Verification items for the finished model (mm, model axes). Give positions to 0.01 mm unless a question says otherwise; leave off trailing zeros. Order: outer loops, then holes, each group sorted by start corner. A loop starts at its lowest first (then second) coordinate and runs counter-clockwise, first axis right, second up. Notation, with made-up numbers: (-29.75, -12.5) -> (-2.75, -12.5) arc R32 ccw to (-2.75, 23.5) -> close; hole circle Ø3 at (13, -16.75). An arc over 180 degrees is marked (long way). Write each question's results on one line, items separated by ' | '. Start each with the question number.
1. Cross-section at B-B, the plane y = -30.5. Enter the section's corners in (x, z), then the cut area to 3 significant figures.
2. Cross-section at A-A, the plane z = 1.45. State how many separate pieces and enclosed holes the cut face has, then the cut area to 3 significant figures.
3. Depth check by flat-ended pin: pin 1 Ø5.5 at (x, y) = (-33.34, 52.39) entering from -Z; pin 2 Ø2.5 at (x, z) = (245, 0.5) entering from -Y; pin 3 Ø1.5 at (x, z) = (4, 0) entering from +Y; pin 4 Ø3 at (y, z) = (19, -0.5) entering from +X. Enter the tip coordinate at first touch or a pass-through.
4. Material ranges on L1, parallel to X at y = 41, z = 1.2 (1 decimal); L2, parallel to X at y = 54.5, z = 1.2 (3 decimals); L3, parallel to X at y = 19.5, z = -1.15, recorded low to high. Write a range as from..to.
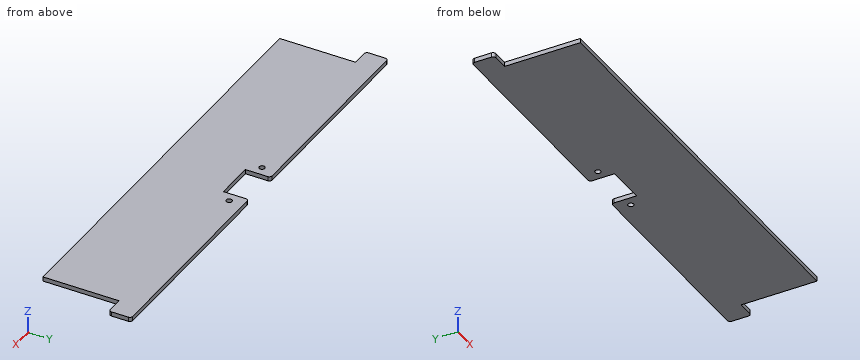
from build123d import *

# Parameters (mm, degrees)
BOSS_EXTRUDE1_DEPTH         = 2.5
SKETCH2_W                   = 44.45
SKETCH2_H                   = 28.575
CUT_EXTRUDE1_DEPTH          = 270.196752221
FILLET1_R                   = 3.175
F_1_4_0_25_DIAMETER_HOLE1_D = 6.35


with BuildPart() as part:
    # Sketch1 → Boss-Extrude1 (new, symmetric)
    with BuildSketch(Plane.XY):
        Polygon((-260.35, 68.2625), (260.35, 68.2625), (260.35, 42.8625), (239.7125, 42.8625), (239.7125, -42.8625), (-239.7125, -42.8625), (-239.7125, 42.8625), (-260.35, 42.8625), align=None)
    extrude(amount=BOSS_EXTRUDE1_DEPTH, both=True)

    # Sketch2 → Cut-Extrude1 (cut, through all)
    with BuildSketch(Plane.XY.offset(2.5)):
        with Locations((0, 53.975)):
            Rectangle(SKETCH2_W, SKETCH2_H)
    extrude(amount=-CUT_EXTRUDE1_DEPTH, mode=Mode.SUBTRACT)

    # Fillet1
    fillet1_edges = [part.edges().sort_by_distance(p)[0] for p in [
        (-260.35, 68.2625, 0),
        (260.35, 68.2625, 0),
        (260.35, 42.8625, 0),
        (-260.35, 42.8625, 0),
        (22.225, 68.2625, 0),
        (-22.225, 68.2625, 0),
    ]]
    fillet(fillet1_edges, radius=FILLET1_R)

    # 1/4 (0.25) Diameter Hole1 (through all)
    with Locations(Plane.XY.offset(2.5)):
        with Locations((-33.3375, 52.3875), (33.3375, 52.3875)):
            Hole(F_1_4_0_25_DIAMETER_HOLE1_D / 2)


solid = part.part
Results below:
1) outline: (-239.71, -2.5) -> (239.71, -2.5) -> (239.71, 2.5) -> (-239.71, 2.5) -> close | area: 2,400 mm²
2) separate pieces: 1 | enclosed holes: 2 | area: 53,000 mm²
3) pin 1: passes through | pin 2: stops at y = 42.86 | pin 3: stops at y = 39.69 | pin 4: stops at x = 239.71
4) L1: x = -239.7..-22.2, 22.2..239.7 | L2: x = -260.35..-35.708, -30.967..-22.225, 22.225..30.967, 35.708..260.35 | L3: x = -239.71..239.71
